The model under review builds one solid part; all positions refer to its coordinate system, in mm. Face numbers are marked on the shaded views. A direction names the side the tool comes from. Coordinates: 2 decimals unless noted, no trailing zeros. Loops run counter-clockwise (first coordinate to the right, second up) from the corner with the lowest first, then second, coordinate; pieces in that order, holes last. Notation, with made-up numbers: M 23,45.25 L 35,45.25 A22 ccw 35,53.25 Z; hole C 49.25,-12.75 d3. An arc over 180 degrees is marked long. Use CSV: the item, a comma, the result in double quotes. Start each with the question number.
from build123d import *

# Parameters (mm, degrees)
SKETCH1_W          = 85.8
SKETCH1_H          = 60
EXTRUDE1_DEPTH     = 30
SKETCH1_5_W        = 10
SKETCH1_5_H        = 12
EXTRUDE2_DEPTH     = 16.5
SKETCH2_R          = 18
SKETCH2_R_2        = 4
EXTRUDE3_DEPTH     = 1.5
SKETCH2_2_R        = 18
SKETCH2_2_R_2      = 4
EXTRUDE4_DEPTH     = 1.5
SKETCH4_R          = 4
EXTRUDE5_DEPTH     = 20.6
SKETCH5_R          = 2.25
CUT_EXTRUDE1_DEPTH = 86
SKETCH6_W          = 10
SKETCH6_H          = 10
CUT_EXTRUDE2_DEPTH = 78.8


with BuildPart() as part:
    # Sketch1 → Extrude1 (new body, symmetric)
    with BuildSketch(Plane.XY):
        with Locations((42.9, 30)):
            Rectangle(SKETCH1_W, SKETCH1_H)
    extrude(amount=EXTRUDE1_DEPTH, both=True)

    # Sketch1<5> → Extrude2 (add, symmetric)
    with BuildSketch(Plane.XY):
        with Locations((5, 66)):
            Rectangle(SKETCH1_5_W, SKETCH1_5_H)
    extrude(amount=EXTRUDE2_DEPTH, both=True)

    # Sketch2 → Extrude3 (add)
    with BuildSketch(Plane(origin=(85.8, 0, 0), x_dir=(0, 0, -1), z_dir=(1, 0, 0))):
        with Locations((0, 30)):
            Circle(SKETCH2_R)
        with Locations((0, 30)):
            Circle(SKETCH2_R_2, mode=Mode.SUBTRACT)
    extrude(amount=EXTRUDE3_DEPTH)

    # Sketch2<2> → Extrude4 (add)
    with BuildSketch(Plane(origin=(85.8, 0, 0), x_dir=(0, 0, -1), z_dir=(1, 0, 0))):
        with Locations((0, 30)):
            Circle(SKETCH2_2_R)
        with Locations((0, 30)):
            Circle(SKETCH2_2_R_2, mode=Mode.SUBTRACT)
    extrude(amount=EXTRUDE4_DEPTH)

    # Sketch4 → Extrude5 (add)
    with BuildSketch(Plane(origin=(85.8, 0, 0), x_dir=(0, 0, -1), z_dir=(1, 0, 0))):
        with Locations((0, 30)):
            Circle(SKETCH4_R)
    extrude(amount=EXTRUDE5_DEPTH)

    # Sketch5 → Cut-Extrude1 (cut)
    with BuildSketch(Plane(origin=(85.8, 0, 0), x_dir=(0, 0, -1), z_dir=(1, 0, 0))):
        with Locations((-25, 55)):
            Circle(SKETCH5_R)
        with Locations((25, 55)):
            Circle(SKETCH5_R)
        with Locations((25, 5)):
            Circle(SKETCH5_R)
        with Locations((-25, 5)):
            Circle(SKETCH5_R)
    extrude(amount=-CUT_EXTRUDE1_DEPTH, mode=Mode.SUBTRACT)

    # Sketch6 → Cut-Extrude2 (cut)
    with BuildSketch(Plane.ZY):
        with Locations((-25, 55)):
            Rectangle(SKETCH6_W, SKETCH6_H)
        with Locations((25, 55)):
            Rectangle(SKETCH6_W, SKETCH6_H)
        with Locations((-25, 5)):
            Rectangle(SKETCH6_W, SKETCH6_H)
        with Locations((25, 5)):
            Rectangle(SKETCH6_W, SKETCH6_H)
    extrude(amount=-CUT_EXTRUDE2_DEPTH, mode=Mode.SUBTRACT)


solid = part.part
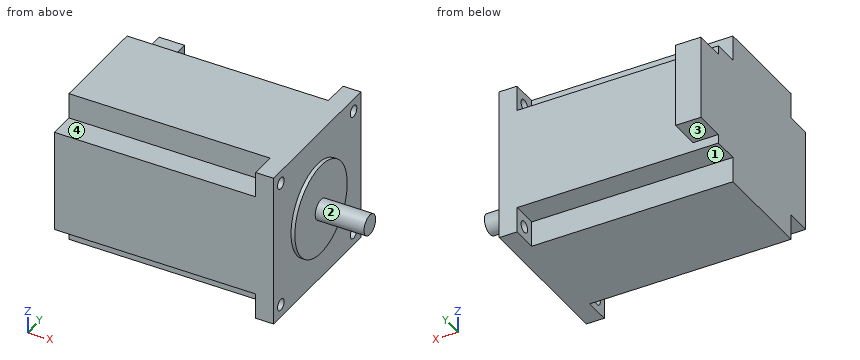
1. Add section D-D (z = 0). Write out the cut boundary in (x, y).
2. Add section C-C (x = 20). Write out the cut boundary in (y, z), plus the area to 3 significant figures.
3. Add section B-B (z = 25). Write out the cut boundary in (x, y), plus the area to 3 significant figures.
4. For the marked faces 1, 2, 3 and 4, list the 3-axis set-ups (+Z, -Z, +X, -X, +Y, -Y) from which the entire face can be reached by the end or side of a thin tool; tool diameter is ignored.
5. Insertion check: pin 1 Ø4 at (x, z) = (89, -12) entering from +Y; pin 2 Ø5 at (x, z) = (59, -24.5) entering from +Y; pin 3 Ø11 at (x, y) = (43.5, 4) entering from -Z. Each pin has a flat end and moves straight along its axis. Give the tip position at first contact, or say it passes through.
6. Add section A-A (y = 55). Write out the cut boundary in (x, z), plus the area to 3 significant figures.
7. To check wall thickness, follow line 1 along Y through (x, z) = (84, -25); line 2 along Y through (x, z) = (48, 24.5); line 3 along Y through (x, z) = (39.5, -17.5). State the ranges of each line that lie inside material, in increasing order.
Solved:
1,outline,"M 0,0 L 85.8,0 L 85.8,12 L 87.3,12 L 87.3,26 L 106.4,26 L 106.4,34 L 87.3,34 L 87.3,48 L 85.8,48 L 85.8,60 L 10,60 L 10,72 L 0,72 Z"
2,outline,"M 0,-20 L 10,-20 L 10,-30 L 50,-30 L 50,-20 L 60,-20 L 60,20 L 50,20 L 50,30 L 10,30 L 10,20 L 0,20 Z"
2,area,"3,200 mm^2"
3,outline,"M 0,10 L 78.8,10 L 78.8,7.25 L 85.8,7.25 L 85.8,52.75 L 78.8,52.75 L 78.8,50 L 0,50 Z; M 78.8,0 L 85.8,0 L 85.8,2.75 L 78.8,2.75 Z; M 78.8,57.25 L 85.8,57.25 L 85.8,60 L 78.8,60 Z"
3,area,"3,510 mm^2"
4,face 1,"-Z, -X, +Y"
4,face 2,"+X"
4,face 3,"-Z, +X, -X, +Y"
4,face 4,"+Z, -X, -Y"
5,pin 1,"stops at y = 44.29"
5,pin 2,"stops at y = 50"
5,pin 3,"stops at z = -20"
6,outline,"M 0,-20 L 78.8,-20 L 78.8,-22.75 L 85.8,-22.75 L 85.8,22.75 L 78.8,22.75 L 78.8,20 L 0,20 Z; M 78.8,-30 L 85.8,-30 L 85.8,-27.25 L 78.8,-27.25 Z; M 78.8,27.25 L 85.8,27.25 L 85.8,30 L 78.8,30 Z"
6,area,"3,510 mm^2"
7,line 1,"y = 0 to 2.75, 7.25 to 52.75, 57.25 to 60"
7,line 2,"y = 10 to 50"
7,line 3,"y = 0 to 60"
